from build123d import *

# Parameters (mm, degrees)
SKETCH1_W           = 101.6
SKETCH1_H           = 101.6
BOSS_EXTRUDE1_DEPTH = 101.6
CHAMFER1_SIZE       = 2.54
SHELL1_T            = 4.7625
CUT_EXTRUDE1_REACH  = 154.4
SKETCH2_R           = 37.5
CUT_EXTRUDE2_REACH  = 126.434
SKETCH3_R           = 3.175


with BuildPart() as part:
    # Sketch1 → Boss-Extrude1 (new body)
    with BuildSketch(Plane(origin=(0, 0, 0), x_dir=(1, 0, 0), z_dir=(0, 1, 0))):
        Rectangle(SKETCH1_W, SKETCH1_H)
    extrude(amount=BOSS_EXTRUDE1_DEPTH)

    # Chamfer1
    chamfer1_edges = [part.edges().sort_by_distance(p)[0] for p in [
        (50.8, 101.6, 0),
        (0, 101.6, -50.8),
        (-50.8, 101.6, 0),
        (0, 0, -50.8),
        (50.8, 0, 0),
        (0, 0, 50.8),
        (-50.8, 0, 0),
        (0, 101.6, 50.8),
        (-50.8, 50.8, -50.8),
        (50.8, 50.8, -50.8),
        (50.8, 50.8, 50.8),
        (-50.8, 50.8, 50.8),
    ]]
    chamfer(chamfer1_edges, length=CHAMFER1_SIZE)

    # Shell1 (no face opened: a closed hollow body)
    add(offset(amount=-SHELL1_T, mode=Mode.PRIVATE), mode=Mode.SUBTRACT)

    # Sketch2 → Cut-Extrude1 (cut, up to next)
    with BuildSketch(Plane.XY.offset(50.8), mode=Mode.PRIVATE) as cut_extrude1_sk1:
        with Locations((0, 50.8)):
            Circle(SKETCH2_R)
    cut_extrude1_tool1 = extrude(cut_extrude1_sk1.sketch, amount=-CUT_EXTRUDE1_REACH, mode=Mode.PRIVATE) & part.part
    add(cut_extrude1_tool1.solids().sort_by_distance((0, 50.8, 50.8))[0], mode=Mode.SUBTRACT)

    # Sketch3 → Cut-Extrude2 (cut, up to next)
    with BuildSketch(Plane(origin=(0, 101.6, 0), x_dir=(1, 0, 0), z_dir=(0, 1, 0)), mode=Mode.PRIVATE) as cut_extrude2_sk1:
        with Locations(Location((-29.21, -29.21, 0), (0, 0, 270))):
            Circle(SKETCH3_R)
    cut_extrude2_tool1 = extrude(cut_extrude2_sk1.sketch, amount=-CUT_EXTRUDE2_REACH, mode=Mode.PRIVATE) & part.part
    # Sketch3 → Cut-Extrude2 (cut, up to next)
    with BuildSketch(Plane(origin=(0, 101.6, 0), x_dir=(1, 0, 0), z_dir=(0, 1, 0)), mode=Mode.PRIVATE) as cut_extrude2_sk2:
        with Locations(Location((29.21, -29.21, 0), (0, 0, 270))):
            Circle(SKETCH3_R)
    cut_extrude2_tool2 = extrude(cut_extrude2_sk2.sketch, amount=-CUT_EXTRUDE2_REACH, mode=Mode.PRIVATE) & part.part
    add(cut_extrude2_tool1.solids().sort_by_distance((-29.21, 101.6, 29.21))[0], mode=Mode.SUBTRACT)
    add(cut_extrude2_tool2.solids().sort_by_distance((29.21, 101.6, 29.21))[0], mode=Mode.SUBTRACT)


solid = part.part
Input: part model. Units: mm. Frame: model coordinates. A direction names the side the tool comes from. Give positions to 0.01 mm unless a question says otherwise; leave off trailing zeros. Order: outer loops, then holes, each group sorted by start corner. A loop starts at its lowest first (then second) coordinate and runs counter-clockwise, first axis right, second up. Notation, with made-up numbers: (56.25, 72) -> (89.25, 72) arc R15 ccw to (89.25, 81) -> close; hole circle Ø4 at (58, 51). An arc over 180 degrees is marked (long way). Use one line per item in the form item = value.
1) Line query: probe 1 along X at (y, z) = (98.2, 29.21) (3 decimals); probe 2 along X at (y, z) = (93.5, -33); probe 3 along X at (y, z) = (99.85, 29.21) (3 decimals). Output: solid intervals per line, ascending.
Response values:
probe_1 = -50.8 to -32.385, -26.035 to 26.035, 32.385 to 50.8
probe_2 = -50.8 to -46.04, 46.04 to 50.8
probe_3 = -50.01 to -32.385, -26.035 to 26.035, 32.385 to 50.01
2) First-contact query: pin 1 Ø8 at (x, y) = (23, 56) entering from +Z; pin 2 Ø5 at (x, z) = (-29.21, 29.21) entering from +Y. Flat tips, straight axial feed; report the tip coordinate or a pass-through.
Response values:
pin_1 = -46.04
pin_2 = 4.76
3) Section C-C, the plane z = 40.5. Return loops of the section in (x, y).
Response values:
outline = (-50.8, 2.54) -> (-48.26, 0) -> (48.26, 0) -> (50.8, 2.54) -> (50.8, 99.06) -> (48.26, 101.6) -> (-48.26, 101.6) -> (-50.8, 99.06) -> close; hole (-46.04, 4.76) -> (46.04, 4.76) -> (46.04, 96.84) -> (-46.04, 96.84) -> close
4) Section A-A, the plane z = 29.21. Return loops of the section in (x, y) (1 decimal).
Response values:
outline = (-50.8, 2.5) -> (-48.3, 0) -> (48.3, 0) -> (50.8, 2.5) -> (50.8, 99.1) -> (48.3, 101.6) -> (32.4, 101.6) -> (32.4, 96.8) -> (46, 96.8) -> (46, 4.8) -> (-46, 4.8) -> (-46, 96.8) -> (-32.4, 96.8) -> (-32.4, 101.6) -> (-48.3, 101.6) -> (-50.8, 99.1) -> close; (-26, 96.8) -> (26, 96.8) -> (26, 101.6) -> (-26, 101.6) -> close
5) Section B-B, the plane y = 90.5. Return loops of the section in (x, z).
Response values:
outline = (-50.8, -48.26) -> (-48.26, -50.8) -> (48.26, -50.8) -> (50.8, -48.26) -> (50.8, 48.26) -> (48.26, 50.8) -> (-48.26, 50.8) -> (-50.8, 48.26) -> close; hole (-46.04, -46.04) -> (46.04, -46.04) -> (46.04, 46.04) -> (-46.04, 46.04) -> close
6) Mould query, pull axis Y, two halves, no side actions, for faces 1 (the cylindrical face through (-4.88, 87.98, 48.45)), 2 (the flat face through (21, 18, 50.8)), 3 (the flat face through (-1, 101.6, -1)). Classes: pulls with the +Y half, pulls with the -Y half, needs draft (parallel to the pull), parting line crosses it, or undercut.
Response values:
face_1 = undercut
face_2 = needs draft
face_3 = pulls with the +Y half
7) Section D-D, the plane x = 10.5. Return loops of the section in (y, z), and give its area (3 significant figures).
Response values:
outline = (0, -48.26) -> (2.54, -50.8) -> (99.06, -50.8) -> (101.6, -48.26) -> (101.6, 48.26) -> (99.06, 50.8) -> (86.8, 50.8) -> (86.8, 46.04) -> (96.84, 46.04) -> (96.84, -46.04) -> (4.76, -46.04) -> (4.76, 46.04) -> (14.8, 46.04) -> (14.8, 50.8) -> (2.54, 50.8) -> (0, 48.26) -> close
area = 1,490 mm^2
8) Reachability of faces 4 (the flat face through (-1, 50, -46.037)), 5 (the cylindrical face through (27.99, 99.25, 32.14)), 6 (the flat face through (-1, 0, -1)) from +Z, -Z, +X, -X, +Y, -Y: full face, straight path, thin tool, end or side. Return the list, or none.
Response values:
face_4 = none
face_5 = +Y
face_6 = +Z, -Z, +X, -X, -Y
